from build123d import *

# Parameters (mm, degrees)
SKETCH4_R                = 28
SKETCH4_R_2              = 25
EXTRUDE_THIN1_DEPTH      = 5
CUT_EXTRUDE1_DEPTH       = 114.247516529
LPATTERN1_COUNT          = 3
LPATTERN1_PITCH          = 10
CIRPATTERN7_COUNT        = 3
CIRPATTERN7_COPY_1_DEPTH = 114.247516529
CIRPATTERN7_COPY_2_DEPTH = 114.247516529
CIRPATTERN7_COPY_3_DEPTH = 114.247516529
CIRPATTERN7_COPY_4_DEPTH = 114.247516529


with BuildPart() as part:
    # Sketch3 → Revolve1 (revolve)
    with BuildSketch(Plane.XY, mode=Mode.PRIVATE) as revolve1_sk:
        with BuildLine():
            Line((0, 0), (0, 100))
            Line((0, 100), (30, 100))
            Line((30, 100), (30, 54.403065089))
            ThreePointArc((30, 54.403065089), (29.682011865, 50.046670749), (28.734788557, 45.782628522))
            Line((28.734788557, 45.782628522), (15, 0))
            Line((15, 0), (0, 0))
        make_face()
    revolve(revolve1_sk.sketch.rotate(Axis((0, 0, 0), (0, 1, 0)), 90), axis=Axis((0, 0, 0), (0, 1, 0)))

    # Sketch4 → Extrude-Thin1 (add)
    with BuildSketch(Plane(origin=(0, 100, 0), x_dir=(1, 0, 0), z_dir=(0, 1, 0))):
        Circle(SKETCH4_R)
        Circle(SKETCH4_R_2, mode=Mode.SUBTRACT)
    extrude(amount=EXTRUDE_THIN1_DEPTH)

    # Sketch9 → Cut-Extrude1 (cut, through all)
    with BuildSketch(Plane.XY):
        with BuildLine():
            Line((-4.256347382, 62.992288971), (5.743652618, 62.992288971))
            ThreePointArc((5.743652618, 62.992288971), (8.243652618, 60.492288971), (5.743652618, 57.992288971))
            Line((5.743652618, 57.992288971), (-4.256347382, 57.992288971))
            ThreePointArc((-4.256347382, 57.992288971), (-6.756347382, 60.492288971), (-4.256347382, 62.992288971))
        make_face()
    cut_extrude1 = extrude(amount=-CUT_EXTRUDE1_DEPTH, mode=Mode.SUBTRACT)

    # LPattern1: Cut-Extrude1 ×3
    with Locations(*[(0, -i * LPATTERN1_PITCH, 0) for i in range(1, LPATTERN1_COUNT)]):
        add(cut_extrude1, mode=Mode.SUBTRACT)

    # CirPattern7: Cut-Extrude1 ×3 about axis
    cirpattern7_axis = Axis((0, 0, 0), (0, -1, 0))
    for i in range(1, CIRPATTERN7_COUNT):
        add(cut_extrude1.rotate(cirpattern7_axis, i * 360 / CIRPATTERN7_COUNT), mode=Mode.SUBTRACT)

    # CirPattern7 copy 1 sketch → CirPattern7 copy 1 (cut, through all)
    with BuildSketch(Plane(origin=(0, -10, 0), x_dir=(-0.4999999999999998, 0, 0.8660254037844387), z_dir=(-0.8660254037844387, 0, -0.4999999999999998))):
        with BuildLine():
            Line((-4.256347382, 62.992288971), (5.743652618, 62.992288971))
            ThreePointArc((5.743652618, 62.992288971), (8.243652618, 60.492288971), (5.743652618, 57.992288971))
            Line((5.743652618, 57.992288971), (-4.256347382, 57.992288971))
            ThreePointArc((-4.256347382, 57.992288971), (-6.756347382, 60.492288971), (-4.256347382, 62.992288971))
        make_face()
    extrude(amount=-CIRPATTERN7_COPY_1_DEPTH, mode=Mode.SUBTRACT)

    # CirPattern7 copy 2 sketch → CirPattern7 copy 2 (cut, through all)
    with BuildSketch(Plane(origin=(0, -10, 0), x_dir=(-0.5000000000000004, 0, -0.8660254037844384), z_dir=(0.8660254037844384, 0, -0.5000000000000004))):
        with BuildLine():
            Line((-4.256347382, 62.992288971), (5.743652618, 62.992288971))
            ThreePointArc((5.743652618, 62.992288971), (8.243652618, 60.492288971), (5.743652618, 57.992288971))
            Line((5.743652618, 57.992288971), (-4.256347382, 57.992288971))
            ThreePointArc((-4.256347382, 57.992288971), (-6.756347382, 60.492288971), (-4.256347382, 62.992288971))
        make_face()
    extrude(amount=-CIRPATTERN7_COPY_2_DEPTH, mode=Mode.SUBTRACT)

    # CirPattern7 copy 3 sketch → CirPattern7 copy 3 (cut, through all)
    with BuildSketch(Plane(origin=(0, -20, 0), x_dir=(-0.4999999999999998, 0, 0.8660254037844387), z_dir=(-0.8660254037844387, 0, -0.4999999999999998))):
        with BuildLine():
            Line((-4.256347382, 62.992288971), (5.743652618, 62.992288971))
            ThreePointArc((5.743652618, 62.992288971), (8.243652618, 60.492288971), (5.743652618, 57.992288971))
            Line((5.743652618, 57.992288971), (-4.256347382, 57.992288971))
            ThreePointArc((-4.256347382, 57.992288971), (-6.756347382, 60.492288971), (-4.256347382, 62.992288971))
        make_face()
    extrude(amount=-CIRPATTERN7_COPY_3_DEPTH, mode=Mode.SUBTRACT)

    # CirPattern7 copy 4 sketch → CirPattern7 copy 4 (cut, through all)
    with BuildSketch(Plane(origin=(0, -20, 0), x_dir=(-0.5000000000000004, 0, -0.8660254037844384), z_dir=(0.8660254037844384, 0, -0.5000000000000004))):
        with BuildLine():
            Line((-4.256347382, 62.992288971), (5.743652618, 62.992288971))
            ThreePointArc((5.743652618, 62.992288971), (8.243652618, 60.492288971), (5.743652618, 57.992288971))
            Line((5.743652618, 57.992288971), (-4.256347382, 57.992288971))
            ThreePointArc((-4.256347382, 57.992288971), (-6.756347382, 60.492288971), (-4.256347382, 62.992288971))
        make_face()
    extrude(amount=-CIRPATTERN7_COPY_4_DEPTH, mode=Mode.SUBTRACT)


solid = part.part
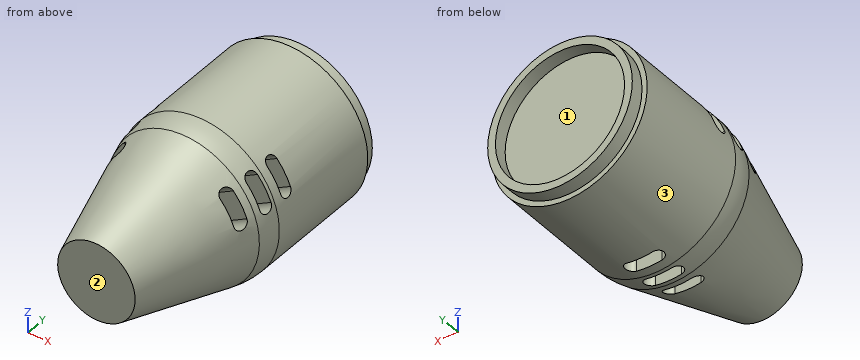
The listing builds one solid part. Answer for the finished solid, in the listing's coordinates (mm). Face numbers are marked on the shaded views. Give positions to 0.01 mm unless a question says otherwise; leave off trailing zeros. Loops run counter-clockwise (first coordinate to the right, second up) from the corner with the lowest first, then second, coordinate; pieces in that order, holes last. Notation, with made-up numbers: (17, 68) - (67, 68) arc R20 cw to (67, 80) - close; hole circle Ø8 at (55, 68.5). An arc over 180 degrees is marked (long way). Use one line per item in the form item = value.
1. Given pin 1 Ø4 at (x, y) = (5.5, 89.5) entering from +Z; pin 2 Ø2 at (x, z) = (-6, 7.5) entering from -Y; pin 3 Ø10 at (y, z) = (86.5, -12) entering from +X; pin 4 Ø4 at (x, z) = (5.5, -6.5) entering from +Y, each flat-ended and moving along its own axis, determine where each tip first touches the part or whether it passes through.
Calculated:
pin_1 = 29.8
pin_2 = 0
pin_3 = 29.17
pin_4 = 100
2. The mould has two halves that part along X. Classify the marked faces 1, 2 and 3: pulls with the +X half, pulls with the -X half, needs draft (parallel to the pull), parting line crosses it, or undercut.
Calculated:
face_1 = undercut
face_2 = needs draft
face_3 = parting line crosses it
3. Section D-D on y = 13.5 is taken. Give the vertices of the cut face in (x, z).
Calculated:
outline = circle Ø38.1 at (0, 0)
4. Section A-A on y = 33 is taken. Give the vertices of the cut face in (x, z).
Calculated:
outline = circle Ø49.8 at (0, 0)
5. Find the intervals of material crossed by line 1 along Y through (x, z) = (6, 6.5); line 2 along Z through (x, y) = (0, 101.8), in increasing order. Write a range as [from, to].
Calculated:
line_1 = [0, 37.99], [42.99, 47.99], [52.99, 57.99], [62.99, 100]
line_2 = [-28, -25], [25, 28]
6. Section B-B on z = 0 is taken. Count the separate pieces of the cut face and the enclosed holes in it, then the cut area to 3 significant figures.
Calculated:
separate_pieces = 1
enclosed_holes = 3
area = 4,860 mm^2
